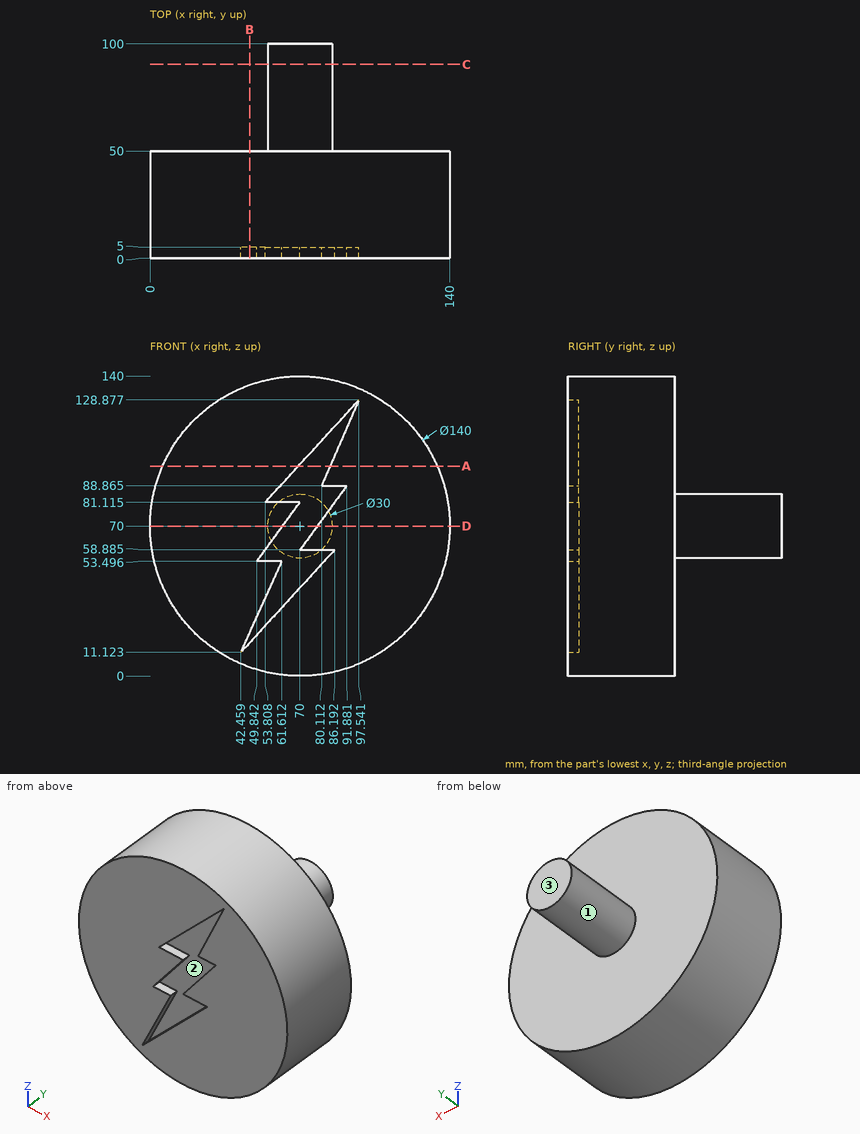
Print and shaded views of the part. All mm, measured from the part's lowest x, y and z. Coordinates: 2 decimals unless noted, no trailing zeros. Loops run counter-clockwise (first coordinate to the right, second up) from the corner with the lowest first, then second, coordinate; pieces in that order, holes last. Notation, with made-up numbers: (-3, 9) - (13, 9) arc R24 ccw to (13, 27) - close; hole circle Ø10 at (3.5, -16.5). An arc over 180 degrees is marked (long way). Use one line per item in the form item = value. Start each with the question number.
1) Band-saw the part on A-A (z = 98). Give the cut face in (x, y), and give its area (3 significant figures).
2) Drill centre lines: L1, parallel to Y at x = 111, z = 81.5; L2, parallel to Z at x = 66.5, y = 89 (1 decimal); L3, parallel to X at y = 19, z = 91 (1 decimal). Where is each one in solid material? Low to high. Write a range as from..to.
3) Band-saw the part on B-B (x = 46.5). Give the cut face in (y, z), and give its area (3 significant figures).
4) Band-saw the part on C-C (y = 90.5). Give the cut face in (x, z), and give its area (3 significant figures).
5) Band-saw the part on D-D (z = 70). Give the cut face in (x, y).
6) Two-plate mould, pull along Z, no slides. Class the marked faces 1, 2 and 3: +Z half, -Z half, draft (parallel to the pull), parting line (faces both ways), or undercut.
7) Flat gauge pins, fed straight in: pin 1 (2 mm diameter, centred on y = 58.5, z = 58, fed in from +X); pin 2 (10 mm diameter, centred on y = 71.5, z = 58, fed in from +X); pin 3 (1.5 mm diameter, centred on x = 58.5, y = 3, fed in from +Z). Where does each tip first touch, or does it go through?
Check values:
q1.outline = (5.84, 0) - (69.27, 0) - (69.27, 5) - (84.09, 5) - (84.09, 0) - (134.16, 0) - (134.16, 50) - (5.84, 50) - close
q1.area = 6,340 mm2
q2.L1 = 0..50
q2.L2 = 55.4..84.6
q2.L3 = 3.2..136.8
q3.outline = (0, 4.06) - (50, 4.06) - (50, 135.94) - (0, 135.94) - (0, 20.06) - (5, 20.06) - (5, 15.54) - (0, 15.54) - close
q3.area = 6,570 mm2
q4.outline = circle Ø30 at (70, 70)
q4.area = 707 mm2
q5.outline = (0, 0) - (61.89, 0) - (61.89, 5) - (78.11, 5) - (78.11, 0) - (140, 0) - (140, 50) - (85, 50) - (85, 100) - (55, 100) - (55, 50) - (0, 50) - close
q6.face_1 = parting line
q6.face_2 = undercut
q6.face_3 = draft
q7.pin_1 = 80.2
q7.pin_2 = 83.27
q7.pin_3 = 139.17
